from build123d import *

# Parameters (mm, degrees)
SKETCH_1_R             = 4
EXTRUDE_1_DEPTH        = 170
HOLE_WIZARD_M4_2_D     = 3.3
HOLE_WIZARD_M4_2_DEPTH = 15.5
HOLE_WIZARD_M4_2_TIP   = 0.991420021


with BuildPart() as part:
    # 草图1 → 凸台-拉伸1 (new body)
    with BuildSketch(Plane.XY):
        Circle(SKETCH_1_R)
    extrude(amount=EXTRUDE_1_DEPTH)

    # 草图5 → M4 螺纹孔1 (revolve, cut)
    with BuildSketch(Plane(origin=(0, 0, 170), x_dir=(0, -1, 0), z_dir=(1, 0, 0))):
        Polygon((0, 0), (0, 16.491420021), (1.65, 15.5), (1.65, 0), align=None)
    revolve(axis=Axis((0, 0, 176.35), (0, 0, -1)), mode=Mode.SUBTRACT)

    # M4 螺纹孔2
    with Locations(Plane(origin=(0, 0, 0), x_dir=(-1, 0, 0), z_dir=(0, 0, -1))):
        with Locations((0, 0)):
            Hole(HOLE_WIZARD_M4_2_D / 2, depth=HOLE_WIZARD_M4_2_DEPTH)
            with Locations((0, 0, -(HOLE_WIZARD_M4_2_DEPTH + HOLE_WIZARD_M4_2_TIP / 2))):  # 118° drill point
                Cone(0, HOLE_WIZARD_M4_2_D / 2, HOLE_WIZARD_M4_2_TIP, mode=Mode.SUBTRACT)


solid = part.part
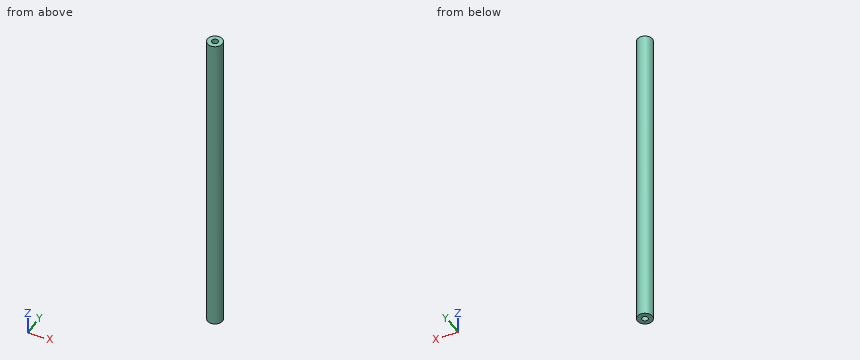
Here's how the part is built. I have some questions about the finished solid (model axes, mm). Give positions to 0.01 mm unless a question says otherwise; leave off trailing zeros. Loops run counter-clockwise (first coordinate to the right, second up) from the corner with the lowest first, then second, coordinate; pieces in that order, holes last. Notation, with made-up numbers: (-8, 16.25) -> (20, 16.25) arc R17 cw to (20, 27.25) -> close; hole circle Ø5 at (-17.5, -25). An arc over 180 degrees is marked (long way). One line per item, written item: value.
Q1. Suppose I cut it at A-A on z = 73. Please give me the cut outline in (x, y).
Answers follow:
outline: circle Ø8 at (0, 0)
Q2. I'm going to push flat-ended pins straight in: pin 1 Ø1.5 at (y, z) = (3, 76) entering from -X; pin 2 Ø1 at (y, z) = (-2.5, 95) entering from -X. Where does each tip first touch, or does it pass through?
Answers follow:
pin 1: x = -3.31
pin 2: x = -3.46
Q3. If I drill on line 1 along Y through (x, z) = (0, 163.75); line 2 along Y through (x, z) = (-1.5, 12.5); line 3 along Y through (x, z) = (0.25, 60.5), over which ranges is the centre line in solid material (lowest first)?
Answers follow:
line 1: -4 to -1.65, 1.65 to 4
line 2: -3.71 to -0.69, 0.69 to 3.71
line 3: -3.99 to 3.99
